from build123d import *

# Parameters (mm, degrees)
SKETCH2_R           = 46
BOSS_EXTRUDE1_DEPTH = 3.175


with BuildPart() as part:
    # Sketch2 → Boss-Extrude1 (new body)
    with BuildSketch(Plane(origin=(0, 0, 0), x_dir=(1, 0, 0), z_dir=(0, 1, 0))):
        Polygon((-50, -16.666666667), (-50, 16.666666667), (-46.825, 16.666666667), (-46.825, 46.825), (-16.666666667, 46.825), (-16.666666667, 50), (16.666666667, 50), (16.666666667, 46.825), (46.825, 46.825), (46.825, 16.666666667), (50, 16.666666667), (50, -16.666666667), (46.825, -16.666666667), (46.825, -46.825), (16.666666667, -46.825), (16.666666667, -50), (-16.666666667, -50), (-16.666666667, -46.825), (-46.825, -46.825), (-46.825, -16.666666667), align=None)
        Circle(SKETCH2_R, mode=Mode.SUBTRACT)
    extrude(amount=BOSS_EXTRUDE1_DEPTH)


solid = part.part
Here's how the part is built. I have some questions about the finished solid (model axes, mm). A direction names the side the tool comes from. Give positions to 0.01 mm unless a question says otherwise; leave off trailing zeros. Order: outer loops, then holes, each group sorted by start corner. A loop starts at its lowest first (then second) coordinate and runs counter-clockwise, first axis right, second up. Notation, with made-up numbers: (70, 76) -> (97, 76) arc R30 ccw to (97, 112) -> close; hole circle Ø9 at (31, 72.5). An arc over 180 degrees is marked (long way). Use a Markdown table: item, result. Add a question column.
Item 1: Imagine slicing it at B-B on y = 2.5. Please give me the cut outline in (x, z) (3 decimals).
Item 2: I need wall thicknesses on line 1 (X direction, y = 0.9, z = 0); line 2 (X direction, y = 0.45, z = -25) (3 decimals). Which ranges of each line are inside material? Lowest first, please.
Item 3: Imagine slicing it at A-A on x = 0. Please give me the cut outline in (y, z) (3 decimals).
Item 4: Will these pins go through, and if not, where does the flat tip stop? pin 1 (1.6 mm diameter, centred on x = -36, y = 1, fed in from -Z) (3 decimals); pin 2 (1 mm diameter, centred on y = 1.5, z = 48.5, fed in from -X); pin 3 (1 mm diameter, centred on y = 2.5, z = 38.5, fed in from +X) (3 decimals).
Item 5: Imagine slicing it at C-C on z = 0. Please give me the cut outline in (x, y) (3 decimals), plus the area to 3 significant figures.
Item 6: For faces 1 (the face through (-16.667, 2, 48)), 2 (the face through (0, 2, 50)), 3 (the face through (16.667, 2, 48)), 4 (the face through (16.667, 2, -48)), 5 (the face through (-46.825, 2, -32)), which set-ups out of +Z, -Z, +X, -X, +Y, -Y let a thin tool reach every point of the face, with its end or its side?
Data:
| question | item | result |
|---|---|---|
| 1 | outline | (-50, -16.667) -> (-46.825, -16.667) -> (-46.825, -46.825) -> (-16.667, -46.825) -> (-16.667, -50) -> (16.667, -50) -> (16.667, -46.825) -> (46.825, -46.825) -> (46.825, -16.667) -> (50, -16.667) -> (50, 16.667) -> (46.825, 16.667) -> (46.825, 46.825) -> (16.667, 46.825) -> (16.667, 50) -> (-16.667, 50) -> (-16.667, 46.825) -> (-46.825, 46.825) -> (-46.825, 16.667) -> (-50, 16.667) -> close; hole circle Ø92 at (0, 0) |
| 2 | line 1 | x = -50 to -46, 46 to 50 |
| 2 | line 2 | x = -46.825 to -38.613, 38.613 to 46.825 |
| 3 | outline | (0, -50) -> (3.175, -50) -> (3.175, -46) -> (0, -46) -> close; (0, 46) -> (3.175, 46) -> (3.175, 50) -> (0, 50) -> close |
| 4 | pin 1 | stops at z = -46.825 |
| 4 | pin 2 | stops at x = -16.67 |
| 4 | pin 3 | stops at x = 46.825 |
| 5 | outline | (-50, 0) -> (-46, 0) -> (-46, 3.175) -> (-50, 3.175) -> close; (46, 0) -> (50, 0) -> (50, 3.175) -> (46, 3.175) -> close |
| 5 | area | 25.4 mm² |
| 6 | face 1 | +Z, -X, +Y, -Y |
| 6 | face 2 | +Z, +X, -X, +Y, -Y |
| 6 | face 3 | +Z, +X, +Y, -Y |
| 6 | face 4 | -Z, +X, +Y, -Y |
| 6 | face 5 | -Z, -X, +Y, -Y |
